```python
from build123d import *

# Parameters (mm, degrees)
AUFSATZ_LINEAR_AUSTRAGEN1_DEPTH = 5
SKIZZE2_W                       = 50.3
SKIZZE2_H                       = 4.8
SCHNITT_LINEAR_AUSTRAGEN1_DEPTH = 5
LINEARES_MUSTER1_COUNT          = 3
LINEARES_MUSTER1_PITCH          = 99.9
SKIZZE3_W                       = 92.912444059
SKIZZE3_H                       = 49.6
SCHNITT_LINEAR_AUSTRAGEN2_DEPTH = 5
LINEARES_MUSTER2_COUNT          = 8
LINEARES_MUSTER2_PITCH          = 99.9
SKIZZE4_W                       = 86.468004991
SKIZZE4_H                       = 49.6
SCHNITT_LINEAR_AUSTRAGEN4_DEPTH = 5
LINEARES_MUSTER3_COUNT          = 7
LINEARES_MUSTER3_PITCH          = 99.9
SKIZZE8_R                       = 40
SCHNITT_LINEAR_AUSTRAGEN5_DEPTH = 10


with BuildPart() as part:
    # Skizze1 → Aufsatz-Linear austragen1 (new body)
    with BuildSketch(Plane.XY):
        with BuildLine():
            Line((0, 0), (0, 700))
            Line((0, 700), (410, 700))
            Line((410, 700), (410, 0))
            Line((410, 0), (370, 0))
            ThreePointArc((370, 0), (355.857864376, 5.857864376), (350, 20))
            Line((350, 20), (350, 80))
            ThreePointArc((350, 80), (344.142135624, 94.142135624), (330, 100))
            Line((330, 100), (80, 100))
            ThreePointArc((80, 100), (65.857864376, 94.142135624), (60, 80))
            Line((60, 80), (60, 20))
            ThreePointArc((60, 20), (54.142135624, 5.857864376), (40, 0))
            Line((40, 0), (0, 0))
        make_face()
    extrude(amount=AUFSATZ_LINEAR_AUSTRAGEN1_DEPTH)

    # Skizze2 → Schnitt-Linear austragen1 (cut)
    with BuildSketch(Plane.XY.offset(5)):
        with Locations((105.1, 202.4)):
            Rectangle(SKIZZE2_W, SKIZZE2_H)
    schnitt_linear_austragen1 = extrude(amount=-SCHNITT_LINEAR_AUSTRAGEN1_DEPTH, mode=Mode.SUBTRACT)

    # Lineares Muster1: Schnitt-Linear austragen1 ×3
    with Locations(*[(i * LINEARES_MUSTER1_PITCH, 0, 0) for i in range(1, LINEARES_MUSTER1_COUNT)]):
        add(schnitt_linear_austragen1, mode=Mode.SUBTRACT)

    # Skizze3 → Schnitt-Linear austragen2 (cut)
    with BuildSketch(Plane.XY.offset(5)):
        with Locations((-41.45622203, 699.3)):
            Rectangle(SKIZZE3_W, SKIZZE3_H)
    schnitt_linear_austragen2 = extrude(amount=-SCHNITT_LINEAR_AUSTRAGEN2_DEPTH, mode=Mode.SUBTRACT)

    # Lineares Muster2: Schnitt-Linear austragen2 ×8
    with Locations(*[(0, -i * LINEARES_MUSTER2_PITCH, 0) for i in range(1, LINEARES_MUSTER2_COUNT)]):
        add(schnitt_linear_austragen2, mode=Mode.SUBTRACT)

    # Skizze4 → Schnitt-Linear austragen4 (cut)
    with BuildSketch(Plane.XY.offset(5)):
        with Locations((448.234002496, 649.7)):
            Rectangle(SKIZZE4_W, SKIZZE4_H)
    schnitt_linear_austragen4 = extrude(amount=-SCHNITT_LINEAR_AUSTRAGEN4_DEPTH, mode=Mode.SUBTRACT)

    # Lineares Muster3: Schnitt-Linear austragen4 ×7
    with Locations(*[(0, -i * LINEARES_MUSTER3_PITCH, 0) for i in range(1, LINEARES_MUSTER3_COUNT)]):
        add(schnitt_linear_austragen4, mode=Mode.SUBTRACT)

    # Skizze8 → Schnitt-Linear austragen5 (cut)
    with BuildSketch(Plane.XY.offset(5)):
        with Locations((335, 274.8)):
            Circle(SKIZZE8_R)
    extrude(amount=-SCHNITT_LINEAR_AUSTRAGEN5_DEPTH, mode=Mode.SUBTRACT)


solid = part.part
```
Input: part model. Units: mm. Frame: model coordinates. A direction names the side the tool comes from. Give positions to 0.01 mm unless a question says otherwise; leave off trailing zeros. Order: outer loops, then holes, each group sorted by start corner. A loop starts at its lowest first (then second) coordinate and runs counter-clockwise, first axis right, second up. Notation, with made-up numbers: M -7.75,64.25 L 28.25,64.25 A13 cw 28.25,85.25 Z; hole C 39.5,-36 d10. An arc over 180 degrees is marked long. Return JSON: item names as keys, results as strings.
1) Section query B-B on x = 317.5. Output: boundary loops of the cut face in (y, z).
Taken from the geometry:
{"outline": "M 100,0 L 200,0 L 200,5 L 100,5 Z; M 204.8,0 L 238.83,0 L 238.83,5 L 204.8,5 Z; M 310.77,0 L 700,0 L 700,5 L 310.77,5 Z"}
2) Access query for faces 3 (the face through (303.26, 250.46, 2.54)), 4 (the face through (356.014, 5.703, 2.465)). Directions: +Z, -Z, +X, -X, +Y, -Y. A direction counts if a zero-diameter tool reaches every point of the face in a straight line with its end or side. Return the directions, or none.
Taken from the geometry:
{"face 3": "+Z, -Z", "face 4": "+Z, -Z, -Y"}
3) Mould query, pull axis X, two halves, no side actions, for faces 1 (the face through (208, 355, 0)), 2 (the face through (66.014, 94.297, 2.465)). Classes: released by +X, released by -X, zero draft, split by the parting line, or undercut.
Taken from the geometry:
{"face 1": "zero draft", "face 2": "undercut"}
4) Section query A-A on x = 220. Output: boundary loops of the cut face in (y, z).
Taken from the geometry:
{"outline": "M 100,0 L 200,0 L 200,5 L 100,5 Z; M 204.8,0 L 700,0 L 700,5 L 204.8,5 Z"}
5) Line query: L1, parallel to Y at x = 328.5, z = 4.05; L2, parallel to Y at x = 219.5, z = 2.3; L3, parallel to Y at x = 332, z = 0.5. Output: solid intervals per line, ascending. Write a range as [from, to].
Taken from the geometry:
{"L1": "y = [100, 200], [204.8, 235.33], [314.27, 700]", "L2": "y = [100, 200], [204.8, 700]", "L3": "y = [99.9, 234.91], [314.69, 700]"}
6) Section query D-D on x = 142.5. Output: boundary loops of the cut face in (y, z).
Taken from the geometry:
{"outline": "M 100,0 L 700,0 L 700,5 L 100,5 Z"}
7) Contact query for flat-ended pins moving along their axis: pin 1 (2 mm diameter, centred on y = 312, z = 3, fed in from -X); pin 2 (1.5 mm diameter, centred on y = 371, z = 2.5, fed in from +X); pin 3 (1.5 mm diameter, centred on x = 1.5, z = 2.5, fed in from -Y); pin 4 (4 mm diameter, centred on x = 346.5, y = 629, fed in from -Z). Output: stop coordinate, or through.
Taken from the geometry:
{"pin 1": "stops at x = 5", "pin 2": "stops at x = 405", "pin 3": "stops at y = 24.8", "pin 4": "stops at z = 0"}
8) Section query C-C on z = 1.1. Count the separate pieces of the cut face and the enclosed holes in it, and give its area (3 significant figures).
Taken from the geometry:
{"separate pieces": "1", "enclosed holes": "4", "area": "249,000 mm2"}
